The drawing under review shows one solid part. Ordinate dimensions are in mm from its lowest x, y, z. Round coordinates to 2 decimals unless told otherwise and drop trailing zeros. Loops run counter-clockwise (first coordinate to the right, second up) from the corner with the lowest first, then second, coordinate; pieces in that order, holes last. Notation, with made-up numbers: (62.25, -0.75) - (103.25, -0.75) arc R22 ccw to (103.25, 32.25) - close; hole circle Ø4 at (17, -33.5). An arc over 180 degrees is marked (long way). Answer as CSV lines item,"result".
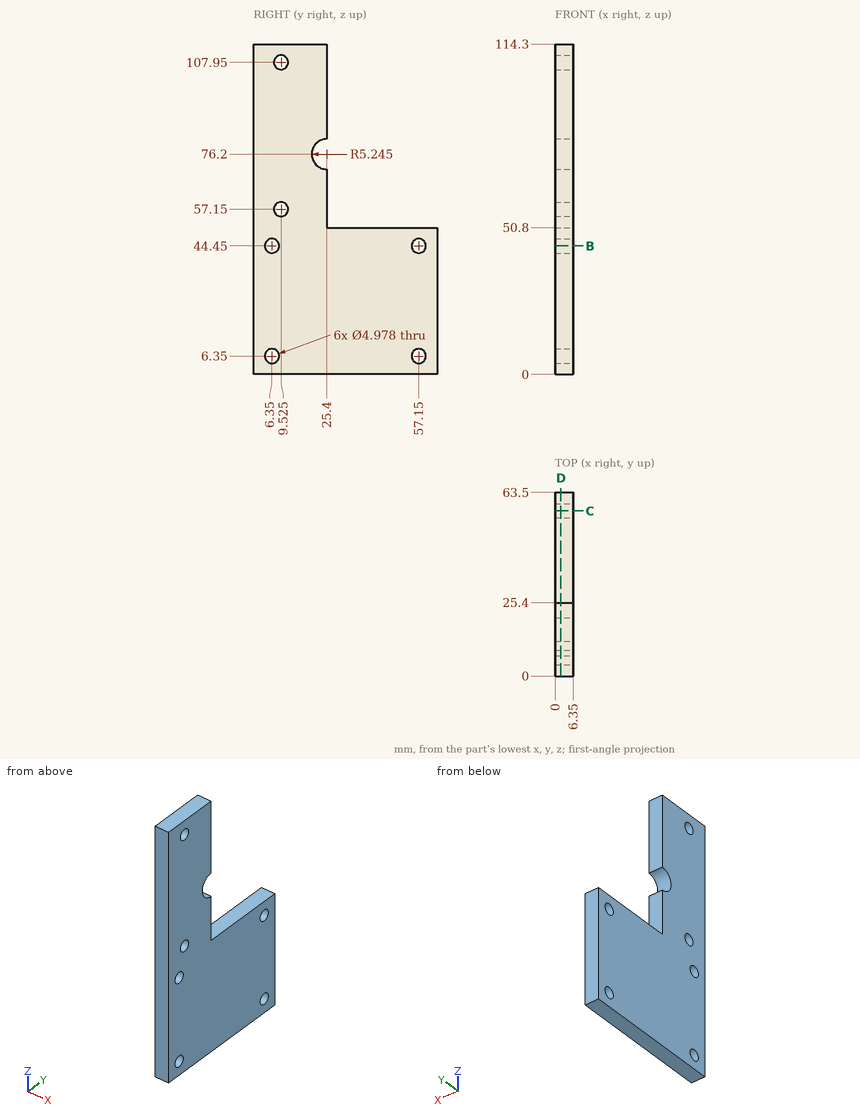
1. Take a section at B-B (z = 44.45). State the section outline as (x, y) points, plus the area to 3 significant figures.
Numbers:
outline,"(0, 0) - (6.35, 0) - (6.35, 3.86) - (0, 3.86) - close; (0, 8.84) - (6.35, 8.84) - (6.35, 54.66) - (0, 54.66) - close; (0, 59.64) - (6.35, 59.64) - (6.35, 63.5) - (0, 63.5) - close"
area,"340 mm²"
2. Wall thickness on probe 1 along Y at (x, z) = (4.5, 44.45); probe 2 along Y at (x, z) = (0.5, 43) (1 decimal); probe 3 along Z at (x, y) = (1.5, 25): over which ranges is each line inside the solid? List them lowest first.
Numbers:
probe 1,"y = 0 to 3.86, 8.84 to 54.66, 59.64 to 63.5"
probe 2,"y = 0 to 4.3, 8.4 to 55.1, 59.2 to 63.5"
probe 3,"z = 0 to 70.97, 81.43 to 114.3"
3. Take a section at D-D (x = 2). State how many separate pieces and enclosed holes the cut face has, plus the area to 3 significant figures.
Numbers:
separate pieces,"1"
enclosed holes,"6"
area,"4,680 mm²"
4. Clearance check with flat-ended pins moving along their axes: pin 1 (1.9 mm diameter, centred on x = 4, z = 105, fed in from +Y); pin 2 (2 mm diameter, centred on x = 4.5, y = 37.5, fed in from -Z). State where each tip first meets the part, or that it passes through.
Numbers:
pin 1,"stops at y = 25.4"
pin 2,"stops at z = 0"
5. Take a section at C-C (y = 57.15). State the section outline as (x, z) points, plus the area to 3 significant figures.
Numbers:
outline,"(0, 0) - (6.35, 0) - (6.35, 3.86) - (0, 3.86) - close; (0, 8.84) - (6.35, 8.84) - (6.35, 41.96) - (0, 41.96) - close; (0, 46.94) - (6.35, 46.94) - (6.35, 50.8) - (0, 50.8) - close"
area,"259 mm²"
